For this review, take the finished solid that the model builds, in its own axes (mm). A direction names the side the tool comes from. Coordinates: 2 decimals unless noted, no trailing zeros. Loops run counter-clockwise (first coordinate to the right, second up) from the corner with the lowest first, then second, coordinate; pieces in that order, holes last. Notation, with made-up numbers: (-27.75, 32.25) - (19.25, 32.25) arc R22 cw to (19.25, 48.25) - close; hole circle Ø9 at (-30.5, -17). An arc over 180 degrees is marked (long way). Answer as a JSON object with one key per item and string values. Group by question number.
Item 1: Clearance check with flat-ended pins moving along their axes: pin 1 (10 mm diameter, centred on x = -12, y = 23, fed in from -Z); pin 2 (8 mm diameter, centred on x = -2.5, y = 15, fed in from -Z); pin 3 (5 mm diameter, centred on x = 0, z = 0, fed in from -Y); pin 4 (10.5 mm diameter, centred on x = 0, y = 22.47, fed in from +Z). State where each tip first meets the part, or that it passes through.
Item 2: Mouldability with a two-part tool opening along Y and no side actions: class faces 1 (the flat face through (7.4, 0, -7.9)), 2 (the cylindrical face through (2.285, 7.998, -3.584)), 3 (the flat face through (0, 40.068, 0)), 4 (the cylindrical face through (-1.277, 16.714, -0.202)) as released by +Y, released by -Y, zero draft, split by the parting line, or undercut.
Item 3: We need section A-A (y = 19). Give the boundary of the cut face in (x, z), then the cut area to 3 significant figures.
Item 4: We need section B-B (y = 5.5). Give the boundary of the cut face in (x, z), then the cut area to 3 significant figures.
Item 5: To check wall thickness, follow line 1 (Y direction, x = 0, z = -8); line 2 (Y direction, x = 2.5, z = -2); line 3 (X direction, y = 22, z = -4). State the ranges of each line that lie inside material, in increasing order.
Item 6: We need section C-C (y = 34). Give the boundary of the cut face in (x, z).
Item 7: Tool access review of faces 5 (the cylindrical face through (-13.725, 23.159, -4.322)), 6 (the flat face through (-2, 3.31, 4)): name each direction out of +Z, -Z, +X, -X, +Y, -Y from which nothing blocks a thin tool from reaching the whole face with its end or side.
from build123d import *

# Parameters (mm, degrees)
CUT_EXTRUDE1_DEPTH         = 47.945551288
CUT_EXTRUDE1_DEPTH_BACK    = 47.945551288
SKETCH2_R                  = 5.8928
M10X1_5_TAPPED_HOLE1_D     = 8.5
M10X1_5_TAPPED_HOLE1_DEPTH = 9.2456
M10X1_5_TAPPED_HOLE1_TIP   = 2.553657631


with BuildPart() as part:
    # Sketch1 → Revolve1 (revolve)
    with BuildSketch(Plane.XY, mode=Mode.PRIVATE) as revolve1_sk:
        Polygon((0, 40.0685), (0, 3.31), (5, 3.31), (10.5974, 0), (17.2974, 0), (14.3891, 15.432044722), (14.3891, 30.672044722), (11.4173, 40.0685), align=None)
    revolve(revolve1_sk.sketch.rotate(Axis((0, 40.0685, 0), (0, -1, 0)), 180), axis=Axis((0, 40.0685, 0), (0, -1, 0)))

    # Sketch2 → Cut-Extrude1 (cut, two sides: drawn at the far end of the back side and taken through both)
    with BuildSketch(Plane.XY.offset(-CUT_EXTRUDE1_DEPTH_BACK)):
        with Locations((0, 22.4663)):
            Circle(SKETCH2_R)
    extrude(amount=CUT_EXTRUDE1_DEPTH + CUT_EXTRUDE1_DEPTH_BACK, mode=Mode.SUBTRACT)

    # M10x1.5 Tapped Hole1
    with Locations(Plane(origin=(0, 3.31, 0), x_dir=(-1, 0, 0), z_dir=(0, -1, 0))):
        with Locations((0, 0)):
            Hole(M10X1_5_TAPPED_HOLE1_D / 2, depth=M10X1_5_TAPPED_HOLE1_DEPTH)
            with Locations((0, 0, -(M10X1_5_TAPPED_HOLE1_DEPTH + M10X1_5_TAPPED_HOLE1_TIP / 2))):  # 118° drill point
                Cone(0, M10X1_5_TAPPED_HOLE1_D / 2, M10X1_5_TAPPED_HOLE1_TIP, mode=Mode.SUBTRACT)


solid = part.part
Check sheet entries:
{
 "1": {"pin 1": "stops at z = -12.57", "pin 2": "stops at z = -15.14", "pin 3": "stops at y = 13.61", "pin 4": "passes through"},
 "2": {"face 1": "released by -Y", "face 2": "zero draft", "face 3": "released by +Y", "face 4": "undercut"},
 "3": {"outline": "(-4.77, -13.58) - (-4.77, 13.58) arc R14.39 ccw to start; (4.77, -13.58) arc R14.39 ccw to (4.77, 13.58) - close", "area": "381 mm2"},
 "4": {"outline": "circle Ø32.52 at (0, 0); hole circle Ø8.5 at (0, 0)", "area": "774 mm2"},
 "5": {"line 1": "y = 1.54 to 16.57, 28.36 to 40.07", "line 2": "y = 13.19 to 17.13, 27.8 to 40.07", "line 3": "x = -13.82 to -5.87, 5.87 to 13.82"},
 "6": {"outline": "circle Ø26.67 at (0, 0)"},
 "7": {"face 5": "+Y", "face 6": "-Y"}
}
